Check sheet for the modelled part. Datum: model origin and axes. Units: mm. A direction names the side the tool comes from. Coordinates: 2 decimals unless noted, no trailing zeros. Write each loop counter-clockwise with the first axis right and the second up, starting at its lowest first coordinate (ties: lowest second). Pieces come first, ordered by that corner, then holes. Notation, with made-up numbers: (24, 85) - (48, 85) arc R27 ccw to (48, 108) - close; hole circle Ø10 at (42, 61). An arc over 180 degrees is marked (long way). Write each question's results on one line, items separated by ' | '.
from build123d import *

# Parameters (mm, degrees)
BOSS_EXTRUDE1_DEPTH = 168


with BuildPart() as part:
    # Sketch1 → Boss-Extrude1 (new body)
    with BuildSketch(Plane(origin=(0, 0, 0), x_dir=(1, 0, 0), z_dir=(0, 1, 0))):
        with BuildLine():
            Line((5.814470124, 4.566536611), (2.829130053, 4.566536611))
            Line((2.829130053, 4.566536611), (2.829130053, -0.01880346))
            ThreePointArc((2.829130053, -0.01880346), (3.703515915, 2.092150748), (5.814470124, 2.966536611))
            Line((5.814470124, 2.966536611), (5.814470124, 4.566536611))
        make_face()
        with BuildLine():
            Line((2.829130053, -0.01880346), (2.829130053, 4.566536611))
            Line((2.829130053, 4.566536611), (-0.185529876, 4.566536611))
            Line((-0.185529876, 4.566536611), (-0.185529876, 2.966536611))
            ThreePointArc((-0.185529876, 2.966536611), (-2.296484085, 2.092150748), (-3.170869947, -0.01880346))
            Line((-3.170869947, -0.01880346), (-3.170869947, -41.433463389))
            Line((-3.170869947, -41.433463389), (2.829130053, -41.433463389))
            Line((2.829130053, -41.433463389), (2.829130053, -0.01880346))
        make_face()
    extrude(amount=BOSS_EXTRUDE1_DEPTH)


solid = part.part
1. Go/stop test with a flat-tipped pin: pin 1 (1 mm diameter, centred on y = 53, z = 16.5, fed in from +X). Record where the tip stops, or that it passes through.
Values follow:
pin 1: stops at x = 2.83
2. Material ranges on L1, parallel to X at y = 105, z = 31; L2, parallel to Z at x = 4.25, y = 110; L3, parallel to Z at x = -1.5, y = 71, recorded low to high. Write a range as [from, to].
Values follow:
L1: x = [-3.17, 2.83] | L2: z = [-4.57, -2.52] | L3: z = [-2.66, 41.43]
3. Sectioned sample at A-A (y = 101). Record the cut outline in (x, z), then the cut area to 3 significant figures.
Values follow:
outline: (-3.17, 0.02) arc R2.99 ccw to (-0.19, -2.97) - (-0.19, -4.57) - (5.81, -4.57) - (5.81, -2.97) arc R2.99 cw to (2.83, 0.02) - (2.83, 41.43) - (-3.17, 41.43) - close | area: 276 mm^2
4. Access from +Z, -Z, +X, -X, +Y, -Y to the whole of each face (thin tool, end or side, straight path). Record for faces 1 (the flat face through (2.829, 83, 21)), 2 (the flat face through (0, 83, 41.433)).
Values follow:
face 1: +Z, +X, +Y, -Y | face 2: +Z, +X, -X, +Y, -Y
5. Sectioned sample at B-B (z = 7.5). Record the cut outline in (x, y).
Values follow:
outline: (-3.17, 0) - (2.83, 0) - (2.83, 168) - (-3.17, 168) - close
